Work out the finished part from the listing and answer in its coordinate system (mm). Coordinates: 2 decimals unless noted, no trailing zeros. Loops run counter-clockwise (first coordinate to the right, second up) from the corner with the lowest first, then second, coordinate; pieces in that order, holes last. Notation, with made-up numbers: (10, 3.5) - (41, 3.5) arc R27 ccw to (41, 39.5) - close; hole circle Ø2 at (60.5, -15.75). An arc over 180 degrees is marked (long way). Write each question's results on one line, items separated by ' | '. Start each with the question number.
1. Find the intervals of material crossed by line 1 along Y through (x, z) = (-12.7, 1.1); line 2 along Y through (x, z) = (-63.5, 0.95) (3 decimals); line 3 along Y through (x, z) = (-35.56, 1.6) (3 decimals), in increasing order. Write a range as [from, to].
2. A cutting plane is placed at B-B on x = -63.5. Determine the outline of the cut face in (y, z) (3 decimals).
3. A cutting plane is placed at A-A on y = 31.75. Determine the outline of the cut face in (x, z) (3 decimals), then the cut area to 3 significant figures.
4. A cutting plane is placed at D-D on x = -35.56. Determine the outline of the cut face in (y, z) (3 decimals).
5. A cutting plane is placed at C-C on z = 1.35. Determine the outline of the cut face in (x, y) (3 decimals), then the cut area to 3 significant figures.
6. Determine the mould class of faces 1 (the flat face through (-39, 101.6, 2)), 2 (the cylindrical face through (-65.646, 91.24, 1.565)), 3 (the flat face through (0, 52, 2)) for opening direction Y: released by +Y, released by -Y, zero draft, split by the parting line, or undercut.
7. Each of these flat-tipped pins is pushed along its axis until it touches: P1, Ø4, axis at x = -35.56, y = 31.75, coming from the +Z side (1 decimal); P2, Ø8, axis at x = -63.5, y = 12.7, coming from the +Z side (3 decimals). Where does it stop, or does it pass through?
Autodesk Inventor part; units mm, degrees
ref_plane "YZ Plane" through (0, 0, 0) normal (1, 0, 0) x (0, 1, 0)
ref_plane "XZ Plane" through (0, 0, 0) normal (0, 1, 0) x (-1, 0, 0)
ref_plane "XY Plane" through (0, 0, 0) normal (0, 0, 1) x (1, 0, 0)
sketch "Sketch1" plane through (0, 0, 0) normal (0, 0, 1) x (1, 0, 0)
  line L0 (0, 0) -> (-76.2, 0)
  line L1 (-76.2, 0) -> (-76.2, 101.6)
  line L2 (-76.2, 101.6) -> (0, 101.6)
  line L3 (0, 101.6) -> (0, 0)
  circle A0 centre (-12.7, 88.9) radius 3.3734
  circle A1 centre (-12.7, 38.1) radius 3.3734
  circle A2 centre (-63.5, 12.7) radius 3.3734
  dimension "d0" = 76.2
  dimension "d1" = 101.6
  dimension "d2" = 6.7469
  dimension "d3" = 12.7
  dimension "d4" = 12.7
  dimension "d5" = 38.1
  dimension "d6" = 12.7
  dimension "d7" = 12.7
  dimension "d8" = 12.7
extrude "Extrusion1" add sketch "Sketch1" along normal blind 3.175
sketch "Sketch2" plane through (0, 0, 3.175) normal (0, 0, 1) x (1, 0, 0)
  line L0 (-76.2, 101.6) -> (-76.2, 0)
  line L1 (-76.2, 101.6) -> (0, 101.6)
  point P0 (0, 0)
  point P1 (-63.5, 88.9)
  point P2 (-35.56, 31.75)
  dimension "d11" = 12.7
  dimension "d12" = 40.64
  dimension "d13" = 12.7
  dimension "d14" = 57.15
hole "Hole1" at (-63.5, 88.9, 3.175) at (-35.56, 31.75, 3.175) direction (0, 0, -1) diameter 6.35 end through all
properties part number "15102898-16-P-0220"
Values:
1) line 1: [0, 34.73], [41.47, 85.53], [92.27, 101.6] | line 2: [0, 9.327], [16.073, 85.725], [92.075, 101.6] | line 3: [0, 28.575], [34.925, 101.6]
2) outline: (0, 0) - (9.327, 0) - (9.327, 3.175) - (0, 3.175) - close; (16.073, 0) - (85.725, 0) - (85.725, 3.175) - (16.073, 3.175) - close; (92.075, 0) - (101.6, 0) - (101.6, 3.175) - (92.075, 3.175) - close
3) outline: (-76.2, 0) - (-38.735, 0) - (-38.735, 3.175) - (-76.2, 3.175) - close; (-32.385, 0) - (0, 0) - (0, 3.175) - (-32.385, 3.175) - close | area: 222 mm^2
4) outline: (0, 0) - (28.575, 0) - (28.575, 3.175) - (0, 3.175) - close; (34.925, 0) - (101.6, 0) - (101.6, 3.175) - (34.925, 3.175) - close
5) outline: (-76.2, 0) - (0, 0) - (0, 101.6) - (-76.2, 101.6) - close; hole circle Ø6.747 at (-63.5, 12.7); hole circle Ø6.35 at (-63.5, 88.9); hole circle Ø6.35 at (-35.56, 31.75); hole circle Ø6.747 at (-12.7, 38.1); hole circle Ø6.747 at (-12.7, 88.9) | area: 7,570 mm^2
6) face 1: released by +Y | face 2: undercut | face 3: zero draft
7) P1: through | P2: z = 3.175
